Autodesk Inventor part; units mm, degrees
ref_plane "YZ Plane" through (0, 0, 0) normal (1, 0, 0) x (0, 1, 0)
ref_plane "XZ Plane" through (0, 0, 0) normal (0, 1, 0) x (-1, 0, 0)
ref_plane "XY Plane" through (0, 0, 0) normal (0, 0, 1) x (1, 0, 0)
sketch "스케치1" plane through (0, 0, 0) normal (0, 1, 0) x (-1, 0, 0)
  line L0 (0, 0) -> (12, 0)
  line L1 (12, 0) -> (12, -4)
  line L2 (12, -4) -> (0, -4)
  line L3 (0, -4) -> (0, 0)
  dimension "d0" = 12
  dimension "d1" = 4
extrude "돌출1" add sketch "스케치1" along normal blind 3
sketch "스케치2" plane through (0, 3, 0) normal (0, 1, 0) x (1, 0, 0)
  line L0 (0, 0) -> (0, 4) construction
  line L1 (0, 2) -> (-12, 2) construction
  line L2 (-12, 4) -> (-12, 0) construction
  point P0 (-1.3, 2)
  point P1 (-7.7, 2)
  point P2 (-10.7, 2)
  dimension "d59" = 1.3
  dimension "d60" = 3
  dimension "d62" = 1.3
hole "구멍1" at (-10.7, 3, -2) at (-1.3, 3, -2) direction (0, -1, 0) diameter 1 end through all
hole "구멍2" at (-7.7, 3, -2) direction (0, -1, 0) diameter 1.6 end through all
equation "\"G23_F\" = 0.65"
equation "\"G23_M\" = 0.67"
equation "\"Screw_F\" = 1.3"
equation "\"Screw_M\" = 1.6"
properties part number "_3D 인쇄"
For this review, take the finished solid that the model builds, in its own axes (mm). Round coordinates to 2 decimals unless told otherwise and drop trailing zeros. Write each loop counter-clockwise with the first axis right and the second up, starting at its lowest first coordinate (ties: lowest second). Pieces come first, ordered by that corner, then holes.
1) Take a section at C-C on y = 1.5. Give the boundary of the cut face in (x, z), then the cut area to 3 significant figures.
Answer below:
outline: (-12, -4) - (0, -4) - (0, 0) - (-12, 0) - close; hole circle Ø1 at (-10.7, -2); hole circle Ø1.6 at (-7.7, -2); hole circle Ø1 at (-1.3, -2)
area: 44.4 mm2
2) Mouldability with a two-part tool opening along X and no side actions: class faces 1 (the face through (-11.196, 1.479, -2.065)), 2 (the face through (0, 1, -2)), 3 (the face through (-6, 0, -2)) as +X half, -X half, draft (parallel to the pull), parting line (faces both ways), or undercut.
Answer below:
face 1: undercut
face 2: +X half
face 3: draft
3) Insertion check: pin 1 Ø1 at (x, z) = (-7.7, -2) entering from -Y. The pin has a flat end and moves straight along its axis. Give the tip position at first contact, or say it passes through.
Answer below:
pin 1: passes through
4) For line 1 along X through (y, z) = (2.35, -2); line 2 along Z through (x, y) = (-10.7, 1.1); line 3 along X through (y, z) = (1.2, -2.4), list the stretches that pass through material, from the lowest coordinate up.
Answer below:
line 1: x = -12 to -11.2, -10.2 to -8.5, -6.9 to -1.8, -0.8 to 0
line 2: z = -4 to -2.5, -1.5 to 0
line 3: x = -12 to -11, -10.4 to -8.39, -7.01 to -1.6, -1 to 0
5) Take a section at D-D on x = -7.7. Give the boundary of the cut face in (y, z), then the cut area to 3 significant figures.
Answer below:
outline: (0, -4) - (3, -4) - (3, -2.8) - (0, -2.8) - close; (0, -1.2) - (3, -1.2) - (3, 0) - (0, 0) - close
area: 7.20 mm2
6) Take a section at B-B on z = -2. Give the boundary of the cut face in (x, y), then the cut area to 3 significant figures.
Answer below:
outline: (-12, 0) - (-11.2, 0) - (-11.2, 3) - (-12, 3) - close; (-10.2, 0) - (-8.5, 0) - (-8.5, 3) - (-10.2, 3) - close; (-6.9, 0) - (-1.8, 0) - (-1.8, 3) - (-6.9, 3) - close; (-0.8, 0) - (0, 0) - (0, 3) - (-0.8, 3) - close
area: 25.2 mm2
7) Take a section at A-A on x = -1.3. Give the boundary of the cut face in (y, z), then the cut area to 3 significant figures.
Answer below:
outline: (0, -4) - (3, -4) - (3, -2.5) - (0, -2.5) - close; (0, -1.5) - (3, -1.5) - (3, 0) - (0, 0) - close
area: 9.00 mm2
